from build123d import *

# Parameters (mm, degrees)
SKETCH1_R           = 160
SKETCH1_R_2         = 1.5
BOSS_EXTRUDE1_DEPTH = 5
CHAMFER1_SIZE       = 1.5


with BuildPart() as part:
    # Sketch1 → Boss-Extrude1 (new body)
    with BuildSketch(Plane(origin=(0, 0, 0), x_dir=(1, 0, 0), z_dir=(0, 1, 0))):
        with Locations(Location((0, 0, 0), (0, 0, 270))):
            Circle(SKETCH1_R)
        with Locations(Location((155, 0, 0), (0, 0, 270))):
            Circle(SKETCH1_R_2, mode=Mode.SUBTRACT)
        with Locations(Location((0, -155, 0), (0, 0, 270))):
            Circle(SKETCH1_R_2, mode=Mode.SUBTRACT)
        with Locations(Location((-155, 0, 0), (0, 0, 270))):
            Circle(SKETCH1_R_2, mode=Mode.SUBTRACT)
        with Locations(Location((0, 155, 0), (0, 0, 270))):
            Circle(SKETCH1_R_2, mode=Mode.SUBTRACT)
    extrude(amount=-BOSS_EXTRUDE1_DEPTH)

    # Chamfer1
    chamfer1_edges = [part.edges().sort_by_distance(p)[0] for p in [
        (-155, 0, -1.5),
        (0, 0, -156.5),
        (155, 0, -1.5),
        (0, 0, 153.5),
    ]]
    chamfer(chamfer1_edges, length=CHAMFER1_SIZE)


solid = part.part
Can you work these out from the model? Positions are in its coordinate system, mm. Give positions to 0.01 mm unless a question says otherwise; leave off trailing zeros. Loops run counter-clockwise (first coordinate to the right, second up) from the corner with the lowest first, then second, coordinate; pieces in that order, holes last. Notation, with made-up numbers: (23, 69.25) -> (47, 69.25) arc R30 cw to (47, 97.25) -> close; hole circle Ø5 at (-24.75, 22.25). An arc over 180 degrees is marked (long way). Use one line per item in the form item = value.
1) If we section it at A-A (y = -4.15): Please give me the cut outline in (x, z), plus the area to 3 significant figures.
Answers:
outline = circle Ø320 at (0, 0); hole circle Ø3 at (-155, 0); hole circle Ø3 at (0, -155); hole circle Ø3 at (0, 155); hole circle Ø3 at (155, 0)
area = 80,400 mm²
2) If we section it at B-B (x = -128): Please give me the cut outline in (y, z), plus the area to 3 significant figures.
Answers:
outline = (-5, -96) -> (0, -96) -> (0, 96) -> (-5, 96) -> close
area = 960 mm²
3) I need wall thicknesses on line 1 along X through (y, z) = (-2.5, 0); line 2 along X through (y, z) = (-4.3, 45); line 3 along X through (y, z) = (-0.4, -2). Which ranges of each line are inside material? Lowest first, please.
Answers:
line_1 = -160 to -156.5, -153.5 to 153.5, 156.5 to 160
line_2 = -153.54 to 153.54
line_3 = -159.99 to -156.66, -153.34 to 153.34, 156.66 to 159.99
4) Will these pins go through, and if not, where does the flat tip stop? pin 1 (2.5 mm diameter, centred on x = 155, z = 0, fed in from -Y); pin 2 (1 mm diameter, centred on y = -3.5, z = 44.5, fed in from -X); pin 3 (6 mm diameter, centred on x = 88, z = 103, fed in from +Y); pin 4 (2 mm diameter, centred on x = -14.5, y = -4.5, fed in from +Z).
Answers:
pin_1 = through
pin_2 = -153.83
pin_3 = 0
pin_4 = 159.43
5) If we section it at C-C (z = 66.5): Please give me the cut outline in (x, y), plus the area to 3 significant figures.
Answers:
outline = (-145.53, -5) -> (145.53, -5) -> (145.53, 0) -> (-145.53, 0) -> close
area = 1,460 mm²
